The listing builds one solid part. Answer for the finished solid, in the listing's coordinates (mm). A direction names the side the tool comes from. Give positions to 0.01 mm unless a question says otherwise; leave off trailing zeros. Write each loop counter-clockwise with the first axis right and the second up, starting at its lowest first coordinate (ties: lowest second). Pieces come first, ordered by that corner, then holes. Notation, with made-up numbers: (15, -15.75) - (71, -15.75) arc R25 cw to (71, 19.25) - close; hole circle Ø11 at (89.25, -23). An arc over 180 degrees is marked (long way). Write each question's results on one line, items separated by ' | '. Start each with the question number.
Q1. For a pull along Z with two mould halves and no side action, classify faces 5 (the face through (-1.99, -90.33, 7.4)), 6 (the face through (-213.843, -9, 26)), 7 (the face through (-144.379, -6.084, 115.742)) as pulls with the +Z half, pulls with the -Z half, needs draft (parallel to the pull), parting line crosses it, or undercut.
Q2. Section C-C (x = 0) is taken. Determine the outline of the cut face in (y, z).
Q3. Flat-ended cylindrical pins translate along their axes: pin 1 Ø3 at (x, z) = (-149.59, 75.25) entering from -Y; pin 2 Ø4 at (x, z) = (102.5, 15) entering from -Y; pin 3 Ø2.5 at (y, z) = (-7, 25.5) entering from +X; pin 4 Ø2.5 at (y, z) = (-7.5, 104.5) entering from -X. Find the tip coordinate at first contact, or state that the pin passes through.
Q4. Section A-A (y = -68) is taken. Determine the outline of the cut face in (x, z), plus the area to 3 significant figures.
Q5. Section B-B (y = -22) is taken. Determine the outline of the cut face in (x, z), plus the area to 3 significant figures.
Q6. For faces 1 (the face through (144.379, -6.084, 115.742)), 2 (the face through (213.843, -9, 106)), 3 (the face through (-205, -6, 130)), 4 (the face through (-141.81, -6.08, 2.15)), determine the directions among +Z, -Z, +X, -X, +Y, -Y from which every point of the face is accessible in a straight line to the end or side of a thin tool.
Q7. Section D-D (y = -101) is taken. Determine the outline of the cut face in (x, z), plus the area to 3 significant figures.
Q8. Find the intervals of material crossed by probe 1 along Z at (x, y) = (223.75, -6); probe 2 along Y at (x, z) = (-203.5, 79); probe 3 along X at (y, z) = (-77, 8), in increasing order.
```python
from build123d import *

# Parameters (mm, degrees)
SKETCH_1_R          = 3.5
EXTRUDE_1_DEPTH     = 15
EXTRUDE_START       = -15
EXTRUDE_2_DEPTH     = 15
CUT_EXTRUDE_1_REACH = 164.969
SKETCH_3_R          = 3.5
EXTRUDE_3_DEPTH     = 12
CUT_EXTRUDE_2_REACH = 287.654
SKETCH_7_R          = 2.5
SKETCH_8_R          = 3
CUT_EXTRUDE_3_DEPTH = 30
CUT_EXTRUDE_4_DEPTH = 4.5
FILLET_1_R          = 5
FILLET_4_R          = 5
FILLET_5_R          = 50
FILLET_6_R          = 50
CUT_EXTRUDE_5_REACH = 287.654
FILLET_7_R          = 10
FILLET_8_R          = 10
FILLET_9_R          = 10
FILLET_10_R         = 10


with BuildPart() as part:
    # Sketch 1 → Extrude 1 (new body)
    with BuildSketch(Plane.XY):
        with BuildLine():
            Line((-110, 0), (-90.35, 0))
            ThreePointArc((-90.35, 0), (0, -90.35), (90.35, 0))
            Line((90.35, 0), (110, 0))
            ThreePointArc((110, 0), (0, -110), (-110, 0))
        make_face()
        with Locations((38.268343237, -92.387953251)):
            Circle(SKETCH_1_R, mode=Mode.SUBTRACT)
        with Locations((-38.268343237, -92.387953251)):
            Circle(SKETCH_1_R, mode=Mode.SUBTRACT)
        with Locations((-92.387953251, -38.268343237)):
            Circle(SKETCH_1_R, mode=Mode.SUBTRACT)
        with Locations((92.387953251, -38.268343237)):
            Circle(SKETCH_1_R, mode=Mode.SUBTRACT)
    extrude(amount=EXTRUDE_1_DEPTH)

    # Sketch 2 → Extrude 2 (add)
    with BuildSketch(Plane.XY.offset(15).offset(EXTRUDE_START)):
        with BuildLine():
            Line((-110, 0), (-129.343495463, 0))
            Line((-129.343495463, 0), (-129.343495463, -12))
            Line((-129.343495463, -12), (-109.343495463, -12))
            ThreePointArc((-109.343495463, -12), (-109.83575124, -6.008972421), (-110, 0))
        make_face()
    extrude_2 = extrude(amount=EXTRUDE_2_DEPTH)

    # Sketch 3 → Cut-Extrude 1 (cut, up to next)
    with BuildSketch(Plane.XZ.offset(12), mode=Mode.PRIVATE) as cut_extrude_1_sk1:
        with Locations((-119.343495463, 7.5)):
            Circle(SKETCH_3_R)
    cut_extrude_1_tool1 = extrude(cut_extrude_1_sk1.sketch, amount=-CUT_EXTRUDE_1_REACH, mode=Mode.PRIVATE) & part.part
    cut_extrude_1 = cut_extrude_1_tool1.solids().sort_by_distance((-119.343495, -12, 7.5))[0]
    add(cut_extrude_1, mode=Mode.SUBTRACT)

    # Mirror 1: Extrude 2, Cut-Extrude 1 across plane
    add(extrude_2.mirror(Plane(origin=(0, 0, 0), x_dir=(0, 0, 1), z_dir=(1, 0, 0))))
    add(cut_extrude_1.mirror(Plane(origin=(0, 0, 0), x_dir=(0, 0, 1), z_dir=(1, 0, 0))), mode=Mode.SUBTRACT)

    # Sketch 4 → Extrude 3 (add)
    with BuildSketch(Plane(origin=(0, 0, 0), x_dir=(1, 0, 0), z_dir=(0, 1, 0))):
        with BuildLine():
            Line((-129.343495463, 0), (-229.343495463, 0))
            Line((-229.343495463, 0), (-229.343495463, -130))
            Line((-229.343495463, -130), (-129.343495463, -130))
            Line((-129.343495463, -130), (-129.343495463, -50))
            ThreePointArc((-129.343495463, -50), (-123.80069115, -29.684939937), (-108.708412194, -15))
            Line((-108.708412194, -15), (-129.343495463, -15))
            Line((-129.343495463, -15), (-129.343495463, 0))
        make_face()
    extrude_3 = extrude(amount=-EXTRUDE_3_DEPTH)

    # Sketch 7 → Cut-Extrude 2 (cut, up to next)
    with BuildSketch(Plane(origin=(0, 0, 0), x_dir=(1, 0, 0), z_dir=(0, 1, 0)), mode=Mode.PRIVATE) as cut_extrude_2_sk1:
        with Locations(Location((-185.657203962, -88.686291501, 0), (0, 0, 270))):
            Circle(SKETCH_7_R)
    cut_extrude_2_tool1 = extrude(cut_extrude_2_sk1.sketch, amount=-CUT_EXTRUDE_2_REACH, mode=Mode.PRIVATE) & part.part
    # Sketch 7 → Cut-Extrude 2 (cut, up to next)
    with BuildSketch(Plane(origin=(0, 0, 0), x_dir=(1, 0, 0), z_dir=(0, 1, 0)), mode=Mode.PRIVATE) as cut_extrude_2_sk2:
        with Locations(Location((-174.343495463, -100, 0), (0, 0, 270))):
            Circle(SKETCH_7_R)
    cut_extrude_2_tool2 = extrude(cut_extrude_2_sk2.sketch, amount=-CUT_EXTRUDE_2_REACH, mode=Mode.PRIVATE) & part.part
    # Sketch 7 → Cut-Extrude 2 (cut, up to next)
    with BuildSketch(Plane(origin=(0, 0, 0), x_dir=(1, 0, 0), z_dir=(0, 1, 0)), mode=Mode.PRIVATE) as cut_extrude_2_sk3:
        with Locations(Location((-160.90846662, -63.937554159, 0), (0, 0, 270))):
            Circle(SKETCH_7_R)
    cut_extrude_2_tool3 = extrude(cut_extrude_2_sk3.sketch, amount=-CUT_EXTRUDE_2_REACH, mode=Mode.PRIVATE) & part.part
    # Sketch 7 → Cut-Extrude 2 (cut, up to next)
    with BuildSketch(Plane(origin=(0, 0, 0), x_dir=(1, 0, 0), z_dir=(0, 1, 0)), mode=Mode.PRIVATE) as cut_extrude_2_sk4:
        with Locations(Location((-149.594758121, -75.251262658, 0), (0, 0, 270))):
            Circle(SKETCH_7_R)
    cut_extrude_2_tool4 = extrude(cut_extrude_2_sk4.sketch, amount=-CUT_EXTRUDE_2_REACH, mode=Mode.PRIVATE) & part.part
    cut_extrude_2_1 = cut_extrude_2_tool1.solids().sort_by_distance((-185.657204, 0, 88.686292))[0]
    add(cut_extrude_2_1, mode=Mode.SUBTRACT)
    cut_extrude_2_2 = cut_extrude_2_tool2.solids().sort_by_distance((-174.343495, 0, 100))[0]
    add(cut_extrude_2_2, mode=Mode.SUBTRACT)
    cut_extrude_2_3 = cut_extrude_2_tool3.solids().sort_by_distance((-160.908467, 0, 63.937554))[0]
    add(cut_extrude_2_3, mode=Mode.SUBTRACT)
    cut_extrude_2_4 = cut_extrude_2_tool4.solids().sort_by_distance((-149.594758, 0, 75.251263))[0]
    add(cut_extrude_2_4, mode=Mode.SUBTRACT)
    cut_extrude_2 = cut_extrude_2_1 + cut_extrude_2_2 + cut_extrude_2_3 + cut_extrude_2_4  # Cut-Extrude 2 as one shape, for the pattern or mirror that repeats it

    # Mirror 2: Extrude 3, Cut-Extrude 2 across plane
    add(extrude_3.mirror(Plane(origin=(0, 0, 0), x_dir=(0, 0, 1), z_dir=(1, 0, 0))))
    add(cut_extrude_2.mirror(Plane(origin=(0, 0, 0), x_dir=(0, 0, 1), z_dir=(1, 0, 0))), mode=Mode.SUBTRACT)

    # Sketch 8 → Cut-Extrude 3 (cut)
    with BuildSketch(Plane.ZY.offset(229.343495463)):
        with Locations((25, -6)):
            Circle(SKETCH_8_R)
        with Locations((105, -6)):
            Circle(SKETCH_8_R)
    cut_extrude_3 = extrude(amount=-CUT_EXTRUDE_3_DEPTH, mode=Mode.SUBTRACT)

    # Sketch 9 → Cut-Extrude 4 (cut)
    with BuildSketch(Plane.ZY.offset(209.343495463)):
        Polygon((20.75, -8.085865128), (20.75, -12), (29.25, -12), (29.25, -8.263652951), (29.25, -3.546261356), (25, -1.092522712), (20.75, -3.546261356), align=None)
        Polygon((109.25, -3.546261356), (105, -1.092522712), (100.75, -3.546261356), (100.75, -8.085865128), (100.75, -12), (109.25, -12), (109.25, -8.263684809), align=None)
    cut_extrude_4 = extrude(amount=CUT_EXTRUDE_4_DEPTH, mode=Mode.SUBTRACT)

    # Fillet 1
    fillet_1_edges = [part.edges().sort_by_distance(p)[0] for p in [
        (-109.343495463, -12, 7.5),
    ]]
    fillet(fillet_1_edges, radius=FILLET_1_R)

    # Fillet 4
    fillet_4_edges = [part.edges().sort_by_distance(p)[0] for p in [
        (109.343495463, -12, 7.5),
    ]]
    fillet(fillet_4_edges, radius=FILLET_4_R)

    # Mirror 4: Cut-Extrude 3, Cut-Extrude 4 across plane
    add(cut_extrude_3.mirror(Plane(origin=(0, 0, 0), x_dir=(0, 0, 1), z_dir=(1, 0, 0))), mode=Mode.SUBTRACT)
    add(cut_extrude_4.mirror(Plane(origin=(0, 0, 0), x_dir=(0, 0, 1), z_dir=(1, 0, 0))), mode=Mode.SUBTRACT)

    # Fillet 5
    fillet_5_edges = [part.edges().sort_by_distance(p)[0] for p in [
        (-129.343495463, -6, 130),
    ]]
    fillet(fillet_5_edges, radius=FILLET_5_R)

    # Fillet 6
    fillet_6_edges = [part.edges().sort_by_distance(p)[0] for p in [
        (129.343495463, -6, 130),
    ]]
    fillet(fillet_6_edges, radius=FILLET_6_R)

    # Sketch 10 → Cut-Extrude 5 (cut, up to next)
    with BuildSketch(Plane(origin=(0, 0, 0), x_dir=(1, 0, 0), z_dir=(0, 1, 0)), mode=Mode.PRIVATE) as cut_extrude_5_sk1:
        with BuildLine():
            Line((-204.343495463, 0), (-144.343495463, 0))
            ThreePointArc((-144.343495463, 0), (-174.343495463, -30), (-204.343495463, 0))
        make_face()
    cut_extrude_5_tool1 = extrude(cut_extrude_5_sk1.sketch, amount=-CUT_EXTRUDE_5_REACH, mode=Mode.PRIVATE) & part.part
    cut_extrude_5 = cut_extrude_5_tool1.solids().sort_by_distance((-174.343495, 0, 12.732395))[0]
    add(cut_extrude_5, mode=Mode.SUBTRACT)

    # Fillet 7
    fillet_7_edges = [part.edges().sort_by_distance(p)[0] for p in [
        (-204.343495463, -6, 0),
    ]]
    fillet(fillet_7_edges, radius=FILLET_7_R)

    # Fillet 8
    fillet_8_edges = [part.edges().sort_by_distance(p)[0] for p in [
        (-144.343495463, -6, 0),
    ]]
    fillet(fillet_8_edges, radius=FILLET_8_R)

    # Mirror 8: Cut-Extrude 5 across plane
    add(cut_extrude_5.mirror(Plane(origin=(0, 0, 0), x_dir=(0, 0, 1), z_dir=(1, 0, 0))), mode=Mode.SUBTRACT)

    # Fillet 9
    fillet_9_edges = [part.edges().sort_by_distance(p)[0] for p in [
        (204.343495463, -6, 0),
    ]]
    fillet(fillet_9_edges, radius=FILLET_9_R)

    # Fillet 10
    fillet_10_edges = [part.edges().sort_by_distance(p)[0] for p in [
        (144.343495463, -6, 0),
    ]]
    fillet(fillet_10_edges, radius=FILLET_10_R)


solid = part.part
```
Answers below:
1) face 5: needs draft | face 6: undercut | face 7: pulls with the +Z half
2) outline: (-110, 0) - (-90.35, 0) - (-90.35, 15) - (-110, 15) - close
3) pin 1: passes through | pin 2: stops at y = -44.72 | pin 3: stops at x = 199.34 | pin 4: stops at x = -199.34
4) outline: (-86.46, 0) - (-59.49, 0) - (-59.49, 15) - (-86.46, 15) - close; (59.49, 0) - (86.46, 0) - (86.46, 15) - (59.49, 15) - close | area: 809 mm2
5) outline: (-107.78, 0) - (-87.63, 0) - (-87.63, 15) - (-107.78, 15) - close; (87.63, 0) - (107.78, 0) - (107.78, 15) - (87.63, 15) - close | area: 604 mm2
6) face 1: +Z, +Y, -Y | face 2: -Y | face 3: +Z, +X, -X, +Y, -Y | face 4: -Z, +Y, -Y
7) outline: (-43.58, 0) - (43.58, 0) - (43.58, 15) - (-43.58, 15) - close | area: 1,310 mm2
8) probe 1: z = 0 to 22, 28 to 102, 108 to 130 | probe 2: y = -12 to 0 | probe 3: x = -78.56 to -47.27, 47.27 to 78.56
